```python
from build123d import *

# Parameters (mm, degrees)
BOSS_EXTRUDE1_DEPTH = 70
BOSS_EXTRUDE2_DEPTH = 2
SKETCH5_R           = 5.5
SKETCH5_R_2         = 1.5
BOSS_EXTRUDE3_DEPTH = 5
SKETCH8_R           = 4.5
CUT_EXTRUDE3_DEPTH  = 5


with BuildPart() as part:
    # Sketch1 → Boss-Extrude1 (new body)
    with BuildSketch(Plane(origin=(0, 0, 0), x_dir=(1, 0, 0), z_dir=(0, 1, 0))):
        with BuildLine():
            Line((-51, 58), (51, 58))
            ThreePointArc((51, 58), (55.949747468, 55.949747468), (58, 51))
            Line((58, 51), (58, -51))
            ThreePointArc((58, -51), (55.949747468, -55.949747468), (51, -58))
            Line((51, -58), (-51, -58))
            ThreePointArc((-51, -58), (-55.949747468, -55.949747468), (-58, -51))
            Line((-58, -51), (-58, 51))
            ThreePointArc((-58, 51), (-55.949747468, 55.949747468), (-51, 58))
        make_face()
        with BuildLine():
            Line((-51, -56), (51, -56))
            ThreePointArc((51, -56), (54.535533906, -54.535533906), (56, -51))
            Line((56, -51), (56, 51))
            ThreePointArc((56, 51), (54.535533906, 54.535533906), (51, 56))
            Line((51, 56), (-51, 56))
            ThreePointArc((-51, 56), (-54.535533906, 54.535533906), (-56, 51))
            Line((-56, 51), (-56, -51))
            ThreePointArc((-56, -51), (-54.535533906, -54.535533906), (-51, -56))
        make_face(mode=Mode.SUBTRACT)
    extrude(amount=BOSS_EXTRUDE1_DEPTH)

    # Sketch3 → Boss-Extrude2 (add)
    with BuildSketch(Plane(origin=(0, 0, 0), x_dir=(1, 0, 0), z_dir=(0, 1, 0))):
        with BuildLine():
            Line((51, 58), (-51, 58))
            ThreePointArc((-51, 58), (-55.949747468, 55.949747468), (-58, 51))
            Line((-58, 51), (-58, -51))
            ThreePointArc((-58, -51), (-55.949747468, -55.949747468), (-51, -58))
            Line((-51, -58), (51, -58))
            ThreePointArc((51, -58), (55.949747468, -55.949747468), (58, -51))
            Line((58, -51), (58, 51))
            ThreePointArc((58, 51), (55.949747468, 55.949747468), (51, 58))
        make_face()
    extrude(amount=BOSS_EXTRUDE2_DEPTH)

    # Sketch5 → Boss-Extrude3 (add)
    with BuildSketch(Plane(origin=(0, 2, 0), x_dir=(1, 0, 0), z_dir=(0, 1, 0))):
        with Locations((-47.5, 47.5)):
            Circle(SKETCH5_R)
        with Locations((-47.5, 47.5)):
            Circle(SKETCH5_R_2, mode=Mode.SUBTRACT)
    extrude(amount=BOSS_EXTRUDE3_DEPTH)

    # Sketch8 → Cut-Extrude3 (cut)
    with BuildSketch(Plane(origin=(0, 0, 0), x_dir=(1, 0, 0), z_dir=(0, 1, 0))):
        with Locations((-47.5, 47.5)):
            Circle(SKETCH8_R)
    extrude(amount=CUT_EXTRUDE3_DEPTH, mode=Mode.SUBTRACT)


solid = part.part
```
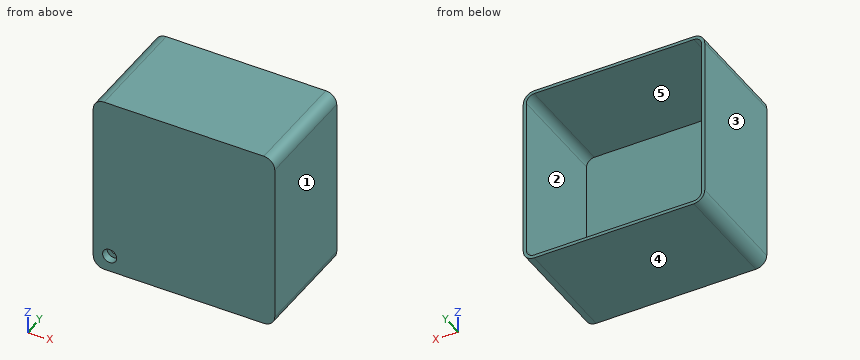
The listing builds one solid part. Answer for the finished solid, in the listing's coordinates (mm). Face numbers are marked on the shaded views. A direction names the side the tool comes from. Round coordinates to 2 decimals unless told otherwise and drop trailing zeros. Loops run counter-clockwise (first coordinate to the right, second up) from the corner with the lowest first, then second, coordinate; pieces in that order, holes last.
Q1. For a pull along X with two mould halves and no side action, classify the marked faces 3, 4 and 5 as released by +X, released by -X, zero draft, split by the parting line, or undercut.
Q2. Section C-C, the plane z = 43 is taken. Determine the outline of the cut face in (x, y).
Q3. Section B-B, the plane z = -47.5 is taken. Determine the outline of the cut face in (x, y).
Q4. Find the intervals of material crossed by line 1 (X direction, y = 6.15, z = -47.5); line 2 (Z direction, x = -47.5, y = 2.45), in increasing order.
Q5. Which of the six approach directions +Z, -Z, +X, -X, +Y, -Y give full straight-line access (tool end or side, diameter ignored) to the marked faces 1 and 2?
Q6. Section A-A, the plane x = -47.5 is taken. Determine the outline of the cut face in (y, z).
Q7. Given pin 1 Ø1 at (x, z) = (16.5, -43) entering from -Y; pin 2 Ø8 at (x, z) = (39.5, 42) entering from +Y; pin 3 Ø5.5 at (x, z) = (-45, -49) entering from +Y; pin 4 Ø4.5 at (x, z) = (-49, -48) entering from -Y, each flat-ended and moving along its own axis, determine where each tip first touches the part or whether it passes through.
Q8. Section D-D, the plane x = -33 is taken. Determine the outline of the cut face in (y, z).
Completed:
1. face 3: released by -X
1. face 4: zero draft
1. face 5: undercut
2. outline: (-58, 0) - (58, 0) - (58, 70) - (56, 70) - (56, 2) - (-56, 2) - (-56, 70) - (-58, 70) - close
3. outline: (-58, 0) - (-52, 0) - (-52, 5) - (-49, 5) - (-49, 7) - (-53, 7) - (-53, 2) - (-56, 2) - (-56, 70) - (-58, 70) - close; (-46, 5) - (-43, 5) - (-43, 0) - (58, 0) - (58, 70) - (56, 70) - (56, 2) - (-42, 2) - (-42, 7) - (-46, 7) - close
4. line 1: x = -58 to -56, -53 to -49, -46 to -42, 56 to 58
4. line 2: z = -58 to -56, -53 to -52, -43 to -42, 56 to 58
5. face 1: +Z, -Z, +X, +Y, -Y
5. face 2: +Y
6. outline: (0, -58) - (70, -58) - (70, -56) - (2, -56) - (2, -53) - (7, -53) - (7, -49) - (5, -49) - (5, -52) - (0, -52) - close; (0, -43) - (5, -43) - (5, -46) - (7, -46) - (7, -42) - (2, -42) - (2, 56) - (70, 56) - (70, 58) - (0, 58) - close
7. pin 1: stops at y = 0
7. pin 2: stops at y = 2
7. pin 3: stops at y = 7
7. pin 4: stops at y = 5
8. outline: (0, -58) - (70, -58) - (70, -56) - (2, -56) - (2, 56) - (70, 56) - (70, 58) - (0, 58) - close
